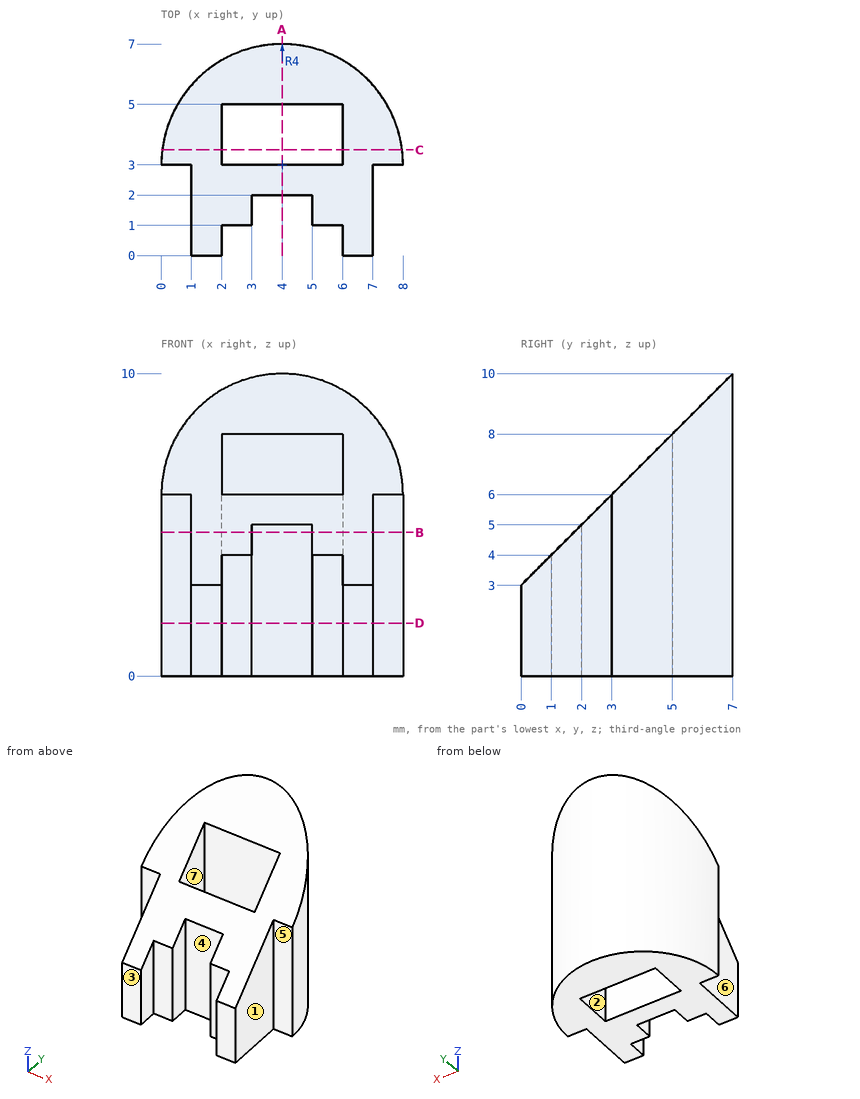
Drawing for the job (mm, zero at the part's lowest x, y, z). A direction names the side the tool comes from. Coordinates: 2 decimals unless noted, no trailing zeros. Write each loop counter-clockwise with the first axis right and the second up, starting at its lowest first coordinate (ties: lowest second). Pieces come first, ordered by that corner, then holes. Notation, with made-up numbers: (37, -7.75) -> (96, -7.75) arc R12 cw to (96, 6.25) -> close; hole circle Ø6 at (-27.75, -33). An arc over 180 degrees is marked (long way). One line per item, written item: value. Start each with the question number.
1) Slice it at A-A on x = 4. Write the cut outline in (y, z).
2) Probe probe 1 along Y at (x, z) = (4, 4.5); probe 2 along X at (y, z) = (4.25, 2.25); probe 3 along Z at (x, y) = (1.25, 4). List the from-to ranges inside material, lowest first.
3) Pull direction X, two halves, no side cores. Call the marked faces 1, 2 and 3: +X half, -X half, draft (parallel to the pull), parting line (faces both ways), or undercut.
4) Slice it at B-B on z = 4.75. Write the cut outline in (x, y).
5) Flat gauge pins, fed straight in: pin 1 Ø1.2 at (x, z) = (4.5, 2.5) entering from -Y; pin 2 Ø1 at (x, z) = (4, 1.5) entering from -Y; pin 3 Ø1 at (y, z) = (4, 5.5) entering from +X. Where does each tip first touch, or does it go through?
6) Slice it at D-D on z = 1.75. Write the cut outline in (x, y), then the cut area to 3 significant figures.
7) Slice it at C-C on y = 3.5. Write the cut outline in (x, z), then the cut area to 3 significant figures.
8) Which spindle directions (+Z, -Z, +X, -X, +Y, -Y) get a long thin tool onto all of the face, cutting with end or side? Do the marked faces 4, 5, 6 and 7. Say none if no direction does.
Answers follow:
1. outline: (2, 0) -> (3, 0) -> (3, 6) -> (2, 5) -> close; (5, 0) -> (7, 0) -> (7, 10) -> (5, 8) -> close
2. probe 1: 2 to 3, 5 to 7
2. probe 2: 0.2 to 2, 6 to 7.8
2. probe 3: 0 to 7
3. face 1: +X half
3. face 2: undercut
3. face 3: draft
4. outline: (0, 3) -> (1, 3) -> (1, 1.75) -> (3, 1.75) -> (3, 2) -> (5, 2) -> (5, 1.75) -> (7, 1.75) -> (7, 3) -> (8, 3) arc R4 ccw to start; hole (2, 3) -> (6, 3) -> (6, 5) -> (2, 5) -> close
5. pin 1: y = 1
5. pin 2: y = 2
5. pin 3: x = 7.97
6. outline: (0, 3) -> (1, 3) -> (1, 0) -> (2, 0) -> (2, 1) -> (3, 1) -> (3, 2) -> (5, 2) -> (5, 1) -> (6, 1) -> (6, 0) -> (7, 0) -> (7, 3) -> (8, 3) arc R4 ccw to start; hole (2, 3) -> (6, 3) -> (6, 5) -> (2, 5) -> close
6. area: 29.1 mm2
7. outline: (0.03, 0) -> (2, 0) -> (2, 6.5) -> (0.03, 6.5) -> close; (6, 0) -> (7.97, 0) -> (7.97, 6.5) -> (6, 6.5) -> close
7. area: 25.6 mm2
8. face 4: +Z, -Z, -Y
8. face 5: +Z, -Z, +X, -Y
8. face 6: +Z, -Z, -X, -Y
8. face 7: +Z, -Z
